from build123d import *

# Parameters (mm, degrees)
F0_R     = 9.109782
F0_W     = 74
F0_H     = 90
F1_DEPTH = 80


with BuildPart() as f1:
    # F0 (on Top) → F1 (new body)
    with BuildSketch(Plane.XY):
        Polygon((608.88648, 650.870509), (-626.11352, 650.870509), (-626.11352, -459.129491), (608.88648, -459.129491), (608.88648, -269.129491), (608.88648, -179.129491), align=None)
        with Locations((-556.11352, -299.129491)):
            Circle(F0_R, mode=Mode.SUBTRACT)
        with Locations((-366.11352, 580.870509)):
            Circle(F0_R, mode=Mode.SUBTRACT)
        with Locations((468.88648, 582.153797)):
            Circle(F0_R, mode=Mode.SUBTRACT)
        with Locations((645.88648, -224.129491)):
            Rectangle(F0_W, F0_H)
        with Locations((652.88648, -224.129491)):
            Circle(F0_R, mode=Mode.SUBTRACT)
    extrude(amount=F1_DEPTH)


solid = f1.part
For this review, take the finished solid that the model builds, in its own axes (mm). A direction names the side the tool comes from. Give positions to 0.01 mm unless a question says otherwise; leave off trailing zeros. Loops run counter-clockwise (first coordinate to the right, second up) from the corner with the lowest first, then second, coordinate; pieces in that order, holes last.
Item 1: For line 1 along X through (y, z) = (336, 24.5); line 2 along Y through (x, z) = (-561, 73.5), list the stretches that pass through material, from the lowest coordinate up.
Item 2: Take a section at A-A, the plane z = 65. State the section outline as (x, y) points, and give its area (3 significant figures).
Item 3: Take a section at B-B, the plane y = 196.5. State the section outline as (x, z) points.
Item 4: Tool access review of faces 1 (the flat face through (608.886, -365, 39)), 2 (the flat face through (608.886, 230, 39)), 3 (the flat face through (682.886, -225, 39)): name each direction out of +Z, -Z, +X, -X, +Y, -Y from which nothing blocks a thin tool from reaching the whole face with its end or side.
Item 5: Insertion check: pin 1 (22 mm diameter, centred on x = 647.5, z = 29.5, fed in from +Y); pin 2 (6 mm diameter, centred on y = -96.5, z = 10, fed in from +X). Each pin has a flat end and moves straight along its axis. Give the tip position at first contact, or say it passes through.
Calculated:
1. line 1: x = -626.11 to 608.89
1. line 2: y = -459.13 to -306.82, -291.44 to 650.87
2. outline: (-626.11, -459.13) - (608.89, -459.13) - (608.89, -269.13) - (682.89, -269.13) - (682.89, -179.13) - (608.89, -179.13) - (608.89, 650.87) - (-626.11, 650.87) - close; hole circle Ø18.22 at (-556.11, -299.13); hole circle Ø18.22 at (-366.11, 580.87); hole circle Ø18.22 at (468.89, 582.15); hole circle Ø18.22 at (652.89, -224.13)
2. area: 1,380,000 mm2
3. outline: (-626.11, 0) - (608.89, 0) - (608.89, 80) - (-626.11, 80) - close
4. face 1: +Z, -Z, +X, -Y
4. face 2: +Z, -Z, +X, +Y
4. face 3: +Z, -Z, +X, +Y, -Y
5. pin 1: stops at y = -179.13
5. pin 2: stops at x = 608.89
